```python
from build123d import *

# Parameters (mm, degrees)
F0_W          = 140
F0_H          = 18
F1_DEPTH      = 85
F0_R          = 9
F0_R_2        = 15
F2_DEPTH      = 12
F3_DEPTH      = 24
F4_DEPTH      = 24
F4_DEPTH_BACK = 12
F5_W          = 140
F5_H          = 49
F5_R          = 8
F6_DEPTH      = 3
F7_DEPTH      = 25


# Not quite as in the source:
# - after a boolean that leaves OpenCascade's solid faulty, fix() repairs it


with BuildPart() as f1:
    # F0 (on Front) → F1 (new body)
    with BuildSketch(Plane.XZ):
        with Locations((0, -9)):
            Rectangle(F0_W, F0_H)
    extrude(amount=F1_DEPTH)

    # F0 (on Front) → F2 (join)
    with BuildSketch(Plane.XZ):
        with BuildLine():
            Line((-70, 38), (-70, 0))
            Line((-70, 0), (70, 0))
            Line((70, 0), (46.8660884819, 105.8705442409))
            ThreePointArc((46.8660884819, 105.8705442409), (47.3410628291, 102.9523352409), (47.5, 100))
            ThreePointArc((47.5, 100), (20, 72.5), (-7.5, 100))
            Line((-7.5, 100), (-7.5, 83))
            ThreePointArc((-7.5, 83), (-14.8223304703, 65.3223304703), (-32.5, 58))
            Line((-32.5, 58), (-50, 58))
            ThreePointArc((-50, 58), (-35.8578643763, 52.1421356237), (-30, 38))
            ThreePointArc((-30, 38), (-50, 18), (-70, 38))
        make_face()
        with BuildLine():
            ThreePointArc((-50, 58), (-64.1421356237, 52.1421356237), (-70, 38))
            ThreePointArc((-70, 38), (-50, 18), (-30, 38))
            ThreePointArc((-30, 38), (-35.8578643763, 52.1421356237), (-50, 58))
        make_face()
        with Locations((-50, 38)):
            Circle(F0_R, mode=Mode.SUBTRACT)
        with BuildLine():
            ThreePointArc((47.5, 100), (47.3410628291, 102.9523352409), (46.8660884819, 105.8705442409))
            ThreePointArc((46.8660884819, 105.8705442409), (17.0476647591, 127.3410628291), (-7.5, 100))
            ThreePointArc((-7.5, 100), (20, 72.5), (47.5, 100))
        make_face()
        with Locations((20, 100)):
            Circle(F0_R_2, mode=Mode.SUBTRACT)
    extrude(amount=F2_DEPTH)

    # F0 (on Front) → F3 (join)
    with BuildSketch(Plane.XZ):
        with BuildLine():
            ThreePointArc((-50, 58), (-64.1421356237, 52.1421356237), (-70, 38))
            ThreePointArc((-70, 38), (-50, 18), (-30, 38))
            ThreePointArc((-30, 38), (-35.8578643763, 52.1421356237), (-50, 58))
        make_face()
        with Locations((-50, 38)):
            Circle(F0_R, mode=Mode.SUBTRACT)
    extrude(amount=F3_DEPTH)

    # F0 (on Front) → F4 (join, two sides)
    with BuildSketch(Plane.XZ) as f4_sk:
        with BuildLine():
            ThreePointArc((47.5, 100), (47.3410628291, 102.9523352409), (46.8660884819, 105.8705442409))
            ThreePointArc((46.8660884819, 105.8705442409), (17.0476647591, 127.3410628291), (-7.5, 100))
            ThreePointArc((-7.5, 100), (20, 72.5), (47.5, 100))
        make_face()
        with Locations((20, 100)):
            Circle(F0_R_2, mode=Mode.SUBTRACT)
    extrude(amount=F4_DEPTH)
    extrude(f4_sk.sketch, amount=-F4_DEPTH_BACK)

    add(f1.part.fix(), mode=Mode.REPLACE)

    # F5 (on face) → F6 (cut)
    with BuildSketch(Plane(origin=(0, 0, -18), x_dir=(1, 0, 0), z_dir=(0, 0, -1))):
        with Locations((0, 42.5)):
            Rectangle(F5_W, F5_H)
        with Locations((-35, 55)):
            Circle(F5_R, mode=Mode.SUBTRACT)
        with Locations((35, 55)):
            Circle(F5_R, mode=Mode.SUBTRACT)
    extrude(amount=-F6_DEPTH, mode=Mode.SUBTRACT)

    # F7 (cut): faces of the model
    f7_faces = [f1.faces().sort_by_distance(p)[0] for p in [
        (-35, -55, -18),
        (35, -55, -18),
    ]]
    extrude(f7_faces, amount=-F7_DEPTH, mode=Mode.SUBTRACT)


solid = f1.part
```
Read the model definition and answer for the solid it produces. Units are mm, in the model's axes. A direction names the side the tool comes from. Coordinates: 2 decimals unless noted, no trailing zeros. Write each loop counter-clockwise with the first axis right and the second up, starting at its lowest first coordinate (ties: lowest second). Pieces come first, ordered by that corner, then holes. Notation, with made-up numbers: (10, 61) -> (22, 61) arc R25 ccw to (22, 73) -> close; hole circle Ø11 at (32.25, 11.25). An arc over 180 degrees is marked (long way). Write item = value, one per line.
(1) Straight lines are drawn through the part: L1, parallel to X at y = -55, z = -6.25; L2, parallel to Z at x = 44.5, y = -36; L3, parallel to Z at x = 20, y = 3.5. For each, find the intervals that lie inside material, in ascending order. Write a range as from..to.
From the geometry:
L1 = -70..-43, -27..27, 43..70
L2 = -15..0
L3 = 72.5..85, 115..127.5
(2) Section B-B on y = -15.5 is taken. Write down the section's boundary in (x, z), plus the area to 3 significant figures.
From the geometry:
outline = (-70, -18) -> (70, -18) -> (70, 0) -> (-70, 0) -> close; circle Ø40 at (-50, 38); circle Ø55 at (20, 100); hole circle Ø18 at (-50, 38); hole circle Ø30 at (20, 100)
area = 5,190 mm2
(3) Section C-C on z = 110 is taken. Write down the section's boundary in (x, y), plus the area to 3 significant figures.
From the geometry:
outline = (-5.62, -24) -> (8.82, -24) -> (8.82, 12) -> (-5.62, 12) -> close; (31.18, -24) -> (45.62, -24) -> (45.62, 12) -> (31.18, 12) -> close
area = 1,040 mm2
(4) Section D-D on y = -51.5 is taken. Write down the section's boundary in (x, z), plus the area to 3 significant figures.
From the geometry:
outline = (-70, -15) -> (-42.19, -15) -> (-42.19, 0) -> (-70, 0) -> close; (-27.81, -15) -> (27.81, -15) -> (27.81, 0) -> (-27.81, 0) -> close; (42.19, -15) -> (70, -15) -> (70, 0) -> (42.19, 0) -> close
area = 1,670 mm2
(5) Section A-A on x = 20 is taken. Write down the section's boundary in (y, z).
From the geometry:
outline = (-85, -18) -> (-67, -18) -> (-67, -15) -> (-18, -15) -> (-18, -18) -> (0, -18) -> (0, 72.5) -> (12, 72.5) -> (12, 85) -> (-24, 85) -> (-24, 72.5) -> (-12, 72.5) -> (-12, 0) -> (-85, 0) -> close; (-24, 115) -> (12, 115) -> (12, 127.5) -> (-24, 127.5) -> close
(6) Given pin 1 Ø9.5 at (x, y) = (35, -55) entering from +Z; pin 2 Ø1.5 at (x, z) = (4, 94.5) entering from -Y; pin 3 Ø1 at (x, z) = (41, 55) entering from -Y; pin 4 Ø3.5 at (x, z) = (-0.5, -16) entering from +Y, each flat-ended and moving along its own axis, determine where each tip first touches the part or whether it passes through.
From the geometry:
pin_1 = through
pin_2 = -24
pin_3 = -12
pin_4 = 0
(7) Which of the six approach directions +Z, -Z, +X, -X, +Y, -Y give full straight-line access (tool end or side, diameter ignored) to faces 5 (the face through (-41, -6, 58)), 6 (the face through (-46, -24, 29)), 7 (the face through (-1, -48, 0)), 8 (the face through (-64.74, -14.5, 51.52))?
From the geometry:
face_5 = +Z, -X, +Y, -Y
face_6 = +Z, +X, -X, -Y
face_7 = +X, -X, -Y
face_8 = -Y
(8) For a pull along Z with two mould halves and no side action, classify faces 1 (the face through (-70, -32, -2)), 2 (the face through (-56.633, -11.832, 44.083)), 3 (the face through (15, -12, 30)), 4 (the face through (-1, -9, -18)) as +Z half, -Z half, draft (parallel to the pull), parting line (faces both ways), or undercut.
From the geometry:
face_1 = draft
face_2 = undercut
face_3 = undercut
face_4 = -Z half
